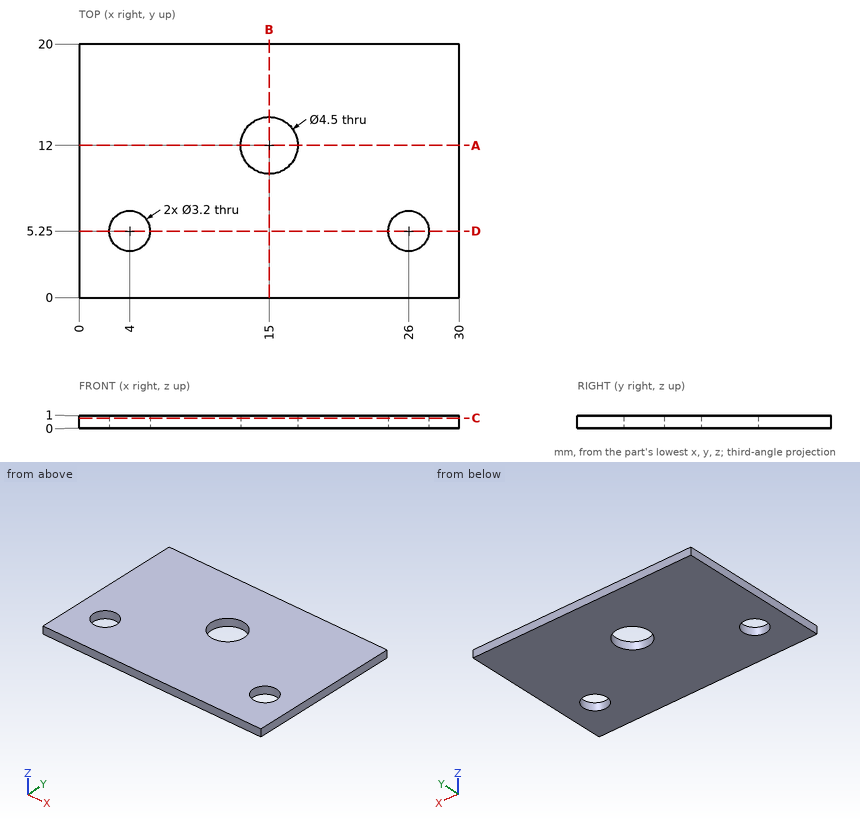
Design review of the part shown in the three views and the two pictorial views. Dimensions are in mm from the part's minimum x, y and z. Coordinates: 2 decimals unless noted, no trailing zeros. Loops run counter-clockwise (first coordinate to the right, second up) from the corner with the lowest first, then second, coordinate; pieces in that order, holes last. Notation, with made-up numbers: M 60,-6.5 L 107,-6.5 A21 ccw 107,10.5 Z; hole C -34.5,-1 d1. An arc over 180 degrees is marked long. Put each result on its own line as item: value. Start each with the question number.
Q1. Wall thickness on line 1 (X direction, y = 5.25, z = 0.7); line 2 (X direction, y = 12, z = 0.65); line 3 (Y direction, x = 4, z = 0.65): over which ranges is each line inside the solid? List them lowest first.
Q2. Add section C-C (z = 0.8). Write out the cut boundary in (x, y).
Q3. Add section D-D (y = 5.25). Write out the cut boundary in (x, z), and give its area (3 significant figures).
Q4. Add section B-B (x = 15). Write out the cut boundary in (y, z).
Q5. Add section A-A (y = 12). Write out the cut boundary in (x, z).
Answers:
1. line 1: x = 0 to 2.4, 5.6 to 24.4, 27.6 to 30
1. line 2: x = 0 to 12.75, 17.25 to 30
1. line 3: y = 0 to 3.65, 6.85 to 20
2. outline: M 0,0 L 30,0 L 30,20 L 0,20 Z; hole C 4,5.25 d3.2; hole C 15,12 d4.5; hole C 26,5.25 d3.2
3. outline: M 0,0 L 2.4,0 L 2.4,1 L 0,1 Z; M 5.6,0 L 24.4,0 L 24.4,1 L 5.6,1 Z; M 27.6,0 L 30,0 L 30,1 L 27.6,1 Z
3. area: 23.6 mm^2
4. outline: M 0,0 L 9.75,0 L 9.75,1 L 0,1 Z; M 14.25,0 L 20,0 L 20,1 L 14.25,1 Z
5. outline: M 0,0 L 12.75,0 L 12.75,1 L 0,1 Z; M 17.25,0 L 30,0 L 30,1 L 17.25,1 Z
